Check sheet for the drawn part. Datum: minimum x, y, z corner. Units: mm. A direction names the side the tool comes from. Give positions to 0.01 mm unless a question says otherwise; leave off trailing zeros. Write each loop counter-clockwise with the first axis right and the second up, starting at its lowest first coordinate (ties: lowest second). Pieces come first, ordered by that corner, then holes. Notation, with made-up numbers: (-13.75, 31) - (33.25, 31) arc R24 cw to (33.25, 44) - close; hole circle Ø10 at (-33.75, 27). An arc over 180 degrees is marked (long way). Return JSON: item names as keys, results as strings. Group by question number.
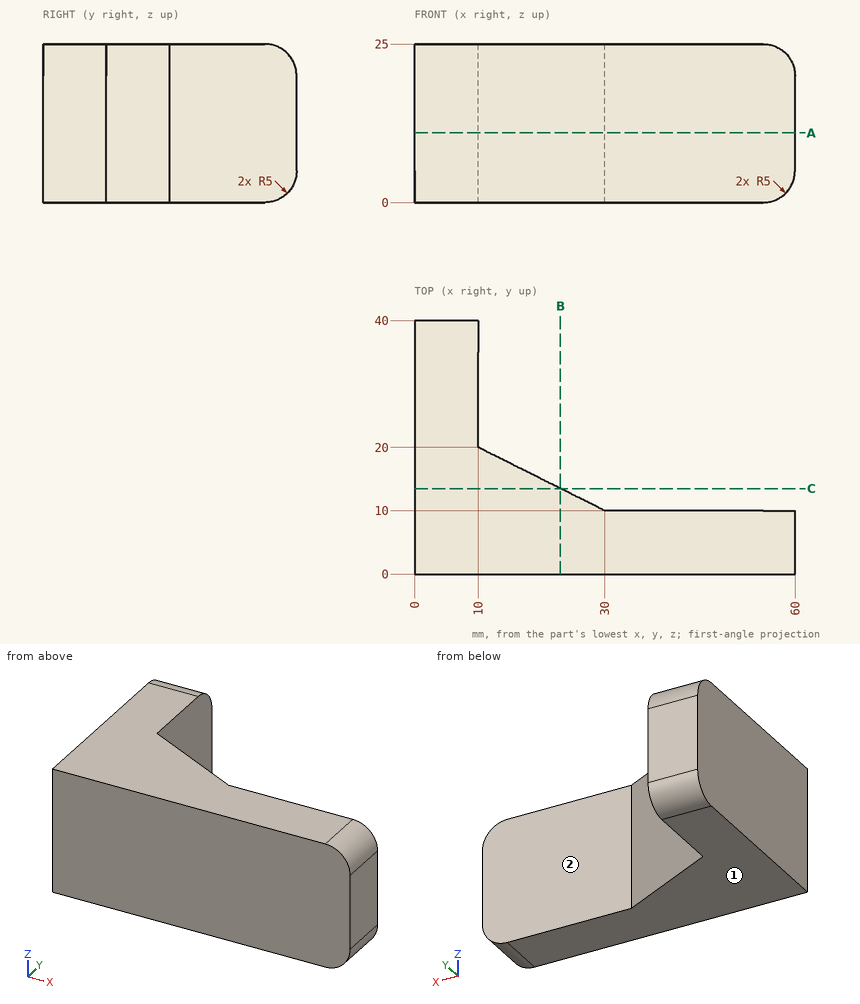
Item 1: Material ranges on line 1 along X through (y, z) = (22, 23); line 2 along X through (y, z) = (12, 10), recorded low to high. Write a range as from..to.
Item 2: Section check B-B on x = 23. Record the cut outline in (y, z), plus the area to 4 significant figures.
Item 3: Depth check by flat-ended pin: pin 1 (1.5 mm diameter, centred on y = 34.5, z = 8.5, fed in from +X); pin 2 (10 mm diameter, centred on x = 41.5, y = 19, fed in from -Z); pin 3 (7.5 mm diameter, centred on x = 42, z = 11, fed in from +Y). Enter the tip coordinate at first touch or a pass-through.
Item 4: Section check C-C on y = 13.5. Record the cut outline in (x, z).
Item 5: Access from +Z, -Z, +X, -X, +Y, -Y to the whole of each face (thin tool, end or side, straight path). Record for the marked faces 1 and 2.
Item 6: Section check A-A on z = 11. Record the cut outline in (x, y), plus the area to 3 significant figures.
Reply:
{
 "1": {"line 1": "0..10", "line 2": "0..26"},
 "2": {"outline": "(0, 0) - (13.5, 0) - (13.5, 25) - (0, 25) - close", "area": "337.5 mm²"},
 "3": {"pin 1": "x = 10", "pin 2": "through", "pin 3": "y = 10"},
 "4": {"outline": "(0, 0) - (23, 0) - (23, 25) - (0, 25) - close"},
 "5": {"face 1": "-Z, +X, -X, +Y, -Y", "face 2": "+Z, -Z, +X, +Y"},
 "6": {"outline": "(0, 0) - (60, 0) - (60, 10) - (30, 10) - (10, 20) - (10, 40) - (0, 40) - close", "area": "1,000 mm²"}
}
